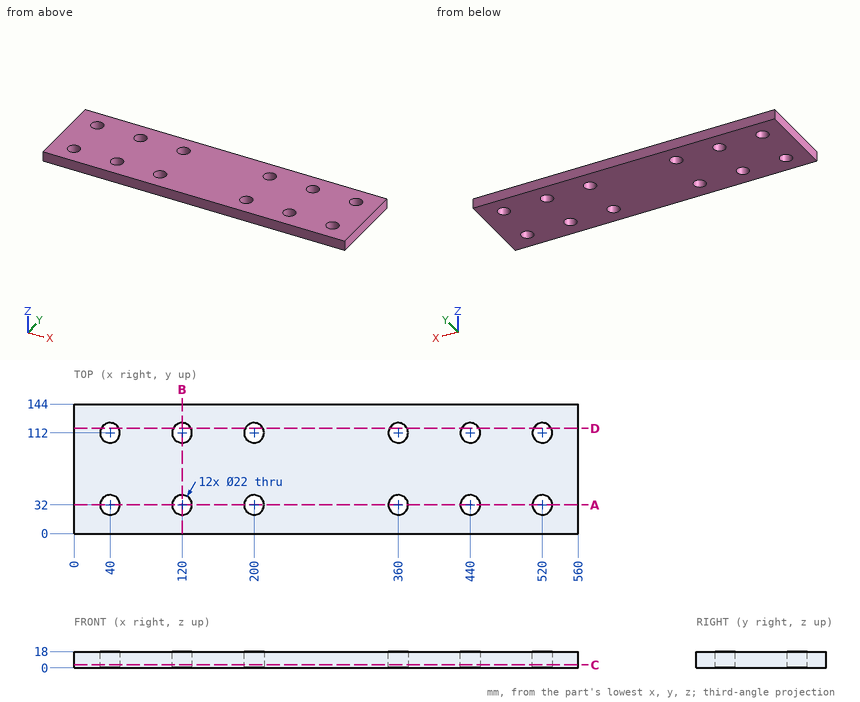
The drawing under review shows one solid part. Ordinate dimensions are in mm from its lowest x, y, z. Coordinates: 2 decimals unless noted, no trailing zeros. Write each loop counter-clockwise with the first axis right and the second up, starting at its lowest first coordinate (ties: lowest second). Pieces come first, ordered by that corner, then holes. Notation, with made-up numbers: M 49,55 L 54,55 A5 cw 54,60 Z; hole C 54,55.25 d9. An arc over 180 degrees is marked long. Put each result on its own line as item: value.
1) Add section C-C on z = 3.25. State how many separate pieces and enclosed holes the cut face has, then the cut area to 3 significant figures.
Computed:
separate pieces: 1
enclosed holes: 12
area: 76,100 mm2
2) Wall thickness on probe 1 along Y at (x, z) = (520, 9.5); probe 2 along Y at (x, z) = (198, 10.75): over which ranges is each line inside the solid? List them lowest first. Write a range as [from, to].
Computed:
probe 1: y = [0, 21], [43, 101], [123, 144]
probe 2: y = [0, 21.18], [42.82, 101.18], [122.82, 144]
3) Add section B-B on x = 120. Give the boundary of the cut face in (y, z), then the cut area to 3 significant figures.
Computed:
outline: M 0,0 L 21,0 L 21,18 L 0,18 Z; M 43,0 L 101,0 L 101,18 L 43,18 Z; M 123,0 L 144,0 L 144,18 L 123,18 Z
area: 1,800 mm2
4) Add section D-D on y = 117. Give the boundary of the cut face in (x, z).
Computed:
outline: M 0,0 L 30.2,0 L 30.2,18 L 0,18 Z; M 49.8,0 L 110.2,0 L 110.2,18 L 49.8,18 Z; M 129.8,0 L 190.2,0 L 190.2,18 L 129.8,18 Z; M 209.8,0 L 350.2,0 L 350.2,18 L 209.8,18 Z; M 369.8,0 L 430.2,0 L 430.2,18 L 369.8,18 Z; M 449.8,0 L 510.2,0 L 510.2,18 L 449.8,18 Z; M 529.8,0 L 560,0 L 560,18 L 529.8,18 Z
5) Add section A-A on y = 32. Give the boundary of the cut face in (x, z).
Computed:
outline: M 0,0 L 29,0 L 29,18 L 0,18 Z; M 51,0 L 109,0 L 109,18 L 51,18 Z; M 131,0 L 189,0 L 189,18 L 131,18 Z; M 211,0 L 349,0 L 349,18 L 211,18 Z; M 371,0 L 429,0 L 429,18 L 371,18 Z; M 451,0 L 509,0 L 509,18 L 451,18 Z; M 531,0 L 560,0 L 560,18 L 531,18 Z
